The listing builds one solid part. Answer for the finished solid, in the listing's coordinates (mm). Face numbers are marked on the shaded views. Give positions to 0.01 mm unless a question says otherwise; leave off trailing zeros. Loops run counter-clockwise (first coordinate to the right, second up) from the corner with the lowest first, then second, coordinate; pieces in that order, holes last. Notation, with made-up numbers: (19.5, -11) - (65.5, -11) arc R9 ccw to (65.5, -4) - close; hole circle Ø6 at (78.25, 74.5). An arc over 180 degrees is marked (long way). Write each question's results on one line, items separated by ' | '.
from build123d import *
from OCP.BRepFilletAPI import BRepFilletAPI_MakeChamfer

# Parameters (mm, degrees)
SKETCH1_W                = 9.5
SKETCH1_H                = 55
BOSS_EXTRUDE1_REACH      = 418.864
BOSS_EXTRUDE1_END_RADIUS = 20
SKETCH2_R                = 15.5
SKETCH2_R_2              = 12.65
BOSS_EXTRUDE2_REACH      = 418.864
BOSS_EXTRUDE2_END_RADIUS = 20
SKETCH3_R                = 15.5
SKETCH3_R_2              = 12.65
SKETCH9_W                = 200
SKETCH9_H                = 33.234380705
CUT_EXTRUDE2_DEPTH       = 198.5
SKETCH8_R                = 18
BOSS_EXTRUDE3_DEPTH      = 15
CHAMFER1_SIZE            = 1
CHAMFER2_SIZE            = 1
CHAMFER2_SIZE2           = 0.883191486
CHAMFER3_SIZE            = 1


with BuildPart() as part:
    # Sketch1 → Revolve1 (revolve)
    with BuildSketch(Plane(origin=(0, 0, 0), x_dir=(1, 0, 0), z_dir=(0, 1, 0)), mode=Mode.PRIVATE) as revolve1_sk:
        with Locations((-4.75, 129.48)):
            Rectangle(SKETCH1_W, SKETCH1_H)
        with Locations((-4.75, -129.48)):
            Rectangle(SKETCH1_W, SKETCH1_H)
    revolve(revolve1_sk.sketch.rotate(Axis((10.5, 0, -101.98), (0, 0, -1)), 180), axis=Axis((10.5, 0, -101.98), (0, 0, -1)))

    # Boss-Extrude1: up to this cylinder (the profile starts outside it)
    boss_extrude1_end = Plane(origin=(10.5, 0, -44.427968), z_dir=(0, 0, 1)) * Cylinder(BOSS_EXTRUDE1_END_RADIUS, 878.728, mode=Mode.PRIVATE)
    # Sketch2 → Boss-Extrude1 (add, up to the surface)
    with BuildSketch(Plane(origin=(-341.54, 0, -30), x_dir=(0.28699849189640086, 0, 0.9579310338689272), z_dir=(-0.9579310338689272, 0, 0.28699849189640086)), mode=Mode.PRIVATE) as boss_extrude1_sk1:
        Circle(SKETCH2_R)
        Circle(SKETCH2_R_2, mode=Mode.SUBTRACT)
    boss_extrude1_tool1 = extrude(boss_extrude1_sk1.sketch, amount=-BOSS_EXTRUDE1_REACH, mode=Mode.PRIVATE) - boss_extrude1_end
    add(boss_extrude1_tool1.solids().sort_by_distance((-345.862655, 0, -44.427968))[0])

    # Boss-Extrude2: up to this cylinder (the profile starts outside it)
    boss_extrude2_end = Plane(origin=(10.5, 0, 15.572032), z_dir=(0, 0, 1)) * Cylinder(BOSS_EXTRUDE2_END_RADIUS, 878.728, mode=Mode.PRIVATE)
    # Sketch3 → Boss-Extrude2 (add, up to the surface)
    with BuildSketch(Plane(origin=(-341.54, 0, 30), x_dir=(-0.28699849189640053, 0, 0.9579310338689273), z_dir=(-0.9579310338689273, 0, -0.28699849189640053)), mode=Mode.PRIVATE) as boss_extrude2_sk1:
        Circle(SKETCH3_R)
        Circle(SKETCH3_R_2, mode=Mode.SUBTRACT)
    boss_extrude2_tool1 = extrude(boss_extrude2_sk1.sketch, amount=-BOSS_EXTRUDE2_REACH, mode=Mode.PRIVATE) - boss_extrude2_end
    add(boss_extrude2_tool1.solids().sort_by_distance((-337.217345, 0, 15.572032))[0])

    # Sketch9 → Cut-Extrude2 (cut, symmetric)
    with BuildSketch(Plane(origin=(-301.587409551, -109.768840106, 0), x_dir=(0, 0, 1), z_dir=(-0.9396926207859128, -0.34202014332565694, 0))):
        with Locations((0, 133.430750104)):
            Rectangle(SKETCH9_W, SKETCH9_H)
    extrude(amount=CUT_EXTRUDE2_DEPTH, both=True, mode=Mode.SUBTRACT)

    # Sketch8 → Boss-Extrude3 (add)
    with BuildSketch(Plane(origin=(-35.886958817, 98.598609003, 0), x_dir=(0, 0, -1), z_dir=(-0.34202014332565694, 0.9396926207859128, 0))):
        with BuildLine():
            Line((-58.125498382, 278.942617703), (58.125498382, 278.942617703))
            Line((58.125498382, 278.942617703), (49.490055464, 338.942617703))
            ThreePointArc((49.490055464, 338.942617703), (0, 381.819808554), (-49.490055464, 338.942617703))
            Line((-49.490055464, 338.942617703), (-58.125498382, 278.942617703))
        make_face()
        with Locations(Location((0, 338.942617703, 0), (0, 0, 90))):
            Circle(SKETCH8_R, mode=Mode.SUBTRACT)
    extrude(amount=BOSS_EXTRUDE3_DEPTH)

    # Chamfer1
    chamfer1_edges = [part.edges().sort_by_distance(p)[0] for p in [
        (-9.5, 0, -156.98),
        (-9.5, 0, -101.98),
        (-9.5, 0, 101.98),
        (-9.5, 0, 156.98),
    ]]
    chamfer(chamfer1_edges, length=CHAMFER1_SIZE)

    # Chamfer2: one chamfer whose edges measure the first distance from different faces: ONE call of the kernel's chamfer builder (chamfer() names one face for all edges)
    chamfer2_edges_1 = [part.edges().sort_by_distance(p)[0] for p in [
        (-298.007278296, 3.194614917, 0),
        (-303.137580446, 17.290004229, 0),
        (-331.328359069, 7.029399929, -53.807776923),
        (-331.328359069, 7.029399929, 53.807776923),
        (-399.810517535, -17.896067331, 0),
        (-329.918850493, -8.420247491, -53.237897301),
        (-329.918850493, -8.420247491, 53.237897301),
        (-394.680215385, -31.991456643, 0),
    ]]
    chamfer2_edges_2 = [part.edges().sort_by_distance(p)[0] for p in [
        (-300.914930544, 11.183323814, -58.125498382),
    ]]
    chamfer2_side_2 = [part.faces().sort_by_distance(p)[0] for p in [
        (-300.973675486, 11.344724214, 0),
    ]]
    chamfer2_edges_3 = [part.edges().sort_by_distance(p)[0] for p in [
        (-300.914930544, 11.183323814, 58.125498382),
    ]]
    chamfer2_side_3 = [part.faces().sort_by_distance(p)[0] for p in [
        (-329.11686309, -0.055580808, 53.758111659),
    ]]
    chamfer2 = BRepFilletAPI_MakeChamfer(part.part.solid().wrapped)
    for e in chamfer2_edges_1:
        chamfer2.Add(CHAMFER2_SIZE, e.wrapped)
    for e in chamfer2_edges_2:
        chamfer2.Add(CHAMFER2_SIZE, CHAMFER2_SIZE2, e.wrapped, chamfer2_side_2[0].wrapped)  # the first distance lies on this face
    for e in chamfer2_edges_3:
        chamfer2.Add(CHAMFER2_SIZE, CHAMFER2_SIZE2, e.wrapped, chamfer2_side_3[0].wrapped)  # the first distance lies on this face
    add(Compound.cast(chamfer2.Shape()), mode=Mode.REPLACE)

    # Chamfer3
    chamfer3_edges = [part.edges().sort_by_distance(p)[0] for p in [
        (-341.07783166, -15.416120436, -28.457394695),
        (-341.07783166, -15.416120436, 28.457394695),
    ]]
    chamfer(chamfer3_edges, length=CHAMFER3_SIZE)


solid = part.part
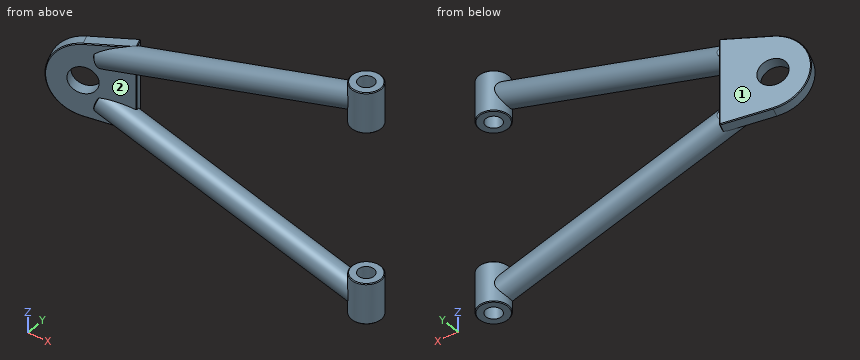
Item 1: Find the intervals of material crossed by line 1 along Y through (x, z) = (10.5, -145); line 2 along Z through (x, y) = (-278, 1); line 3 along Z through (x, y) = (-79.5, -13.5), in increasing order. Write a range as [from, to].
Values found:
line 1: y = [-20, -10.5], [10.5, 20] | line 2: z = [-65.18, -62.2], [-35.87, -32.89], [32.89, 35.87], [62.2, 65.18] | line 3: z = [-116.46, -100.56], [100.56, 116.46]
Item 2: For a pull along Z with two mould halves and no side action, classify the marked faces 1 and 2 as released by +Z, released by -Z, zero draft, split by the parting line, or undercut.
Values found:
face 1: zero draft | face 2: undercut
Item 3: A cutting plane is placed at B-B, the plane z = 125.5. Count the separate pieces of the cut face and the enclosed holes in it, plus the area to 3 significant figures.
Values found:
separate pieces: 1 | enclosed holes: 2 | area: 1,460 mm²
Item 4: A cutting plane is placed at A-A, the plane x = 10.5. Determine the outline of the cut face in (y, z).
Values found:
outline: (-20, -155.98) - (-19, -156.98) - (-10.5, -156.98) - (-10.5, -101.98) - (-19, -101.98) - (-20, -102.98) - close; (-20, 102.98) - (-19, 101.98) - (-10.5, 101.98) - (-10.5, 156.98) - (-19, 156.98) - (-20, 155.98) - close; (10.5, -156.98) - (19, -156.98) - (20, -155.98) - (20, -102.98) - (19, -101.98) - (10.5, -101.98) - close; (10.5, 101.98) - (19, 101.98) - (20, 102.98) - (20, 155.98) - (19, 156.98) - (10.5, 156.98) - close
Item 5: Flat-ended cylindrical pins translate along their axes: P1, Ø4, axis at x = -296.5, y = 4.5, coming from the -Z side; P2, Ø4, axis at x = -150, z = 75, coming from the -Y side; P3, Ø2, axis at y = -13, z = -117.5, coming from the +X side. Find the tip coordinate at first contact, or state that the pin passes through.
Values found:
P1: stops at z = -59.78 | P2: stops at y = -11.96 | P3: stops at x = 26.5
